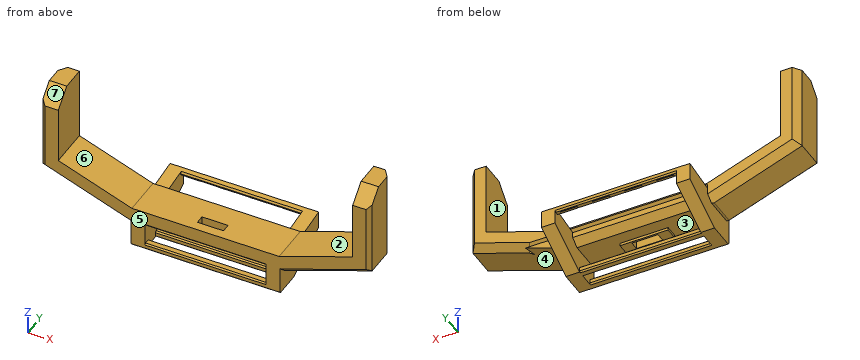
```python
from build123d import *
from OCP.BRepFilletAPI import BRepFilletAPI_MakeChamfer

# Parameters (mm, degrees)
BOSS_EXTRUDE1_DEPTH      = 300
CHAMFER1_SIZE            = 30
CHAMFER2_SIZE            = 120
BOSS_EXTRUDE2_DEPTH      = 180
BOSS_EXTRUDE2_DEPTH_BACK = 120
SKETCH3_W                = 101.940118113
SKETCH3_H                = 551.842685694
CUT_EXTRUDE7_DEPTH       = 1991.965553697
CHAMFER3_SIZE            = 170
CHAMFER3_SIZE2           = 348.551653068
SKETCH6_W                = 46.442322401
SKETCH6_H                = 54.989404456
SKETCH6_H_2              = 57.655849519
BOSS_EXTRUDE3_DEPTH      = 906.440509715
CHAMFER5_SIZE            = 10
CHAMFER5_SIZE2           = 11.720638091
SKETCH7_W                = 359.809632682
SKETCH7_H                = 90.64577865
BOSS_EXTRUDE4_DEPTH      = 20
SKETCH8_W                = 195
SKETCH8_H                = 65
CUT_EXTRUDE8_DEPTH       = 392
SKETCH9_W                = 124.341085276
SKETCH9_H                = 16.237188454
BOSS_EXTRUDE5_DEPTH      = 5
CHAMFER6_SIZE            = 60
CHAMFER6_SIZE2           = 43.59255168


with BuildPart() as part:
    # Sketch2 → Boss-Extrude1 (new body)
    with BuildSketch(Plane(origin=(0, 0, 0), x_dir=(1, 0, 0), z_dir=(0, 1, 0))):
        Polygon((-1100, -366.154475502), (-1100, 177.470675031), (-550, 377.470675031), (550, 377.470675031), (1100, 177.470675031), (1100, -377.470675031), (1230, -377.470675031), (1230, 268.52621943), (572.902747098, 507.470675031), (-572.902747098, 507.470675031), (-1230, 268.52621943), (-1230, -366.154475502), align=None)
    extrude(amount=BOSS_EXTRUDE1_DEPTH)

    # Chamfer1
    chamfer1_edges = [part.edges().sort_by_distance(p)[0] for p in [
        (-1230, 0, 48.814128036),
        (-901.451373549, 0, -387.99844723),
        (0, 0, -507.470675031),
        (901.451373549, 0, -387.99844723),
        (1230, 0, 54.4722278),
    ]]
    chamfer(chamfer1_edges, length=CHAMFER1_SIZE)

    # Chamfer2
    chamfer2_edges = [part.edges().sort_by_distance(p)[0] for p in [
        (-1150, 0, 366.154475502),
        (1150, 0, 377.470675031),
    ]]
    chamfer(chamfer2_edges, length=CHAMFER2_SIZE)

    # Sketch3 → Boss-Extrude2 (add, two sides: drawn at the far end of the back side and taken through both)
    with BuildSketch(Plane(origin=(0, 0, -507.470675031), x_dir=(-1, 0, 0), z_dir=(0, 0, -1)).offset(-BOSS_EXTRUDE2_DEPTH_BACK)):
        with Locations((-504.190313915, 275.921342847)):
            Rectangle(SKETCH3_W, SKETCH3_H)
        with Locations((504.190313915, 275.921342847)):
            Rectangle(SKETCH3_W, SKETCH3_H)
    extrude(amount=BOSS_EXTRUDE2_DEPTH + BOSS_EXTRUDE2_DEPTH_BACK)

    # Sketch5 → Cut-Extrude7 (cut, through all)
    with BuildSketch(Plane.ZY.offset(555.160372971)):
        Polygon((-387.470675031, 551.842685694), (-433.497227826, 219.864084998), (-387.470675031, 300), align=None)
    extrude(amount=-CUT_EXTRUDE7_DEPTH, mode=Mode.SUBTRACT)

    # Chamfer3: one chamfer whose edges measure the first distance from different faces: ONE call of the kernel's chamfer builder (chamfer() names one face for all edges)
    chamfer3_edges_1 = [part.edges().sort_by_distance(p)[0] for p in [
        (-504.190313915, 551.842685694, -687.470675031),
    ]]
    chamfer3_side_1 = [part.faces().sort_by_distance(p)[0] for p in [
        (-504.190313915, 551.842685694, -537.470675031),
    ]]
    chamfer3_edges_2 = [part.edges().sort_by_distance(p)[0] for p in [
        (504.190313915, 551.842685694, -687.470675031),
    ]]
    chamfer3_side_2 = [part.faces().sort_by_distance(p)[0] for p in [
        (504.190313915, 551.842685694, -537.470675031),
    ]]
    chamfer3 = BRepFilletAPI_MakeChamfer(part.part.solid().wrapped)
    for e in chamfer3_edges_1:
        chamfer3.Add(CHAMFER3_SIZE, CHAMFER3_SIZE2, e.wrapped, chamfer3_side_1[0].wrapped)  # the first distance lies on this face
    for e in chamfer3_edges_2:
        chamfer3.Add(CHAMFER3_SIZE, CHAMFER3_SIZE2, e.wrapped, chamfer3_side_2[0].wrapped)  # the first distance lies on this face
    add(Compound.cast(chamfer3.Shape()), mode=Mode.REPLACE)

    # Sketch6 → Boss-Extrude3 (add)
    with BuildSketch(Plane(origin=(-453.220254858, 0, 0), x_dir=(0, 0, -1), z_dir=(1, 0, 0))):
        Polygon((387.470675031, 551.842685694), (393.758008235, 506.493643621), (421.699837769, 506.493643621), (421.699837769, 551.842685694), align=None)
        with Locations((664.249513831, 175.796330397)):
            Rectangle(SKETCH6_W, SKETCH6_H)
        with Locations((664.249513831, 28.82792476)):
            Rectangle(SKETCH6_W, SKETCH6_H_2)
    extrude(amount=BOSS_EXTRUDE3_DEPTH)

    # Chamfer5: one chamfer whose edges measure the first distance from different faces: ONE call of the kernel's chamfer builder (chamfer() names one face for all edges)
    chamfer5_edges_1 = [part.edges().sort_by_distance(p)[0] for p in [
        (0, 506.493643621, -421.699837769),
        (0, 551.842685694, -421.699837769),
        (0, 148.301628169, -641.02835263),
        (0, 203.291032625, -641.02835263),
        (0, 203.291032625, -687.470675031),
        (0, 148.301628169, -687.470675031),
        (0, 0, -641.02835263),
        (0, 57.655849519, -641.02835263),
        (0, 57.655849519, -687.470675031),
        (0, 0, -687.470675031),
    ]]
    chamfer5_edges_2 = [part.edges().sort_by_distance(p)[0] for p in [
        (0, 506.493643621, -393.758008235),
    ]]
    chamfer5_side_2 = [part.faces().sort_by_distance(p)[0] for p in [
        (-541.133646758, 425.921342847, -404.928804327),
    ]]
    chamfer5 = BRepFilletAPI_MakeChamfer(part.part.solid().wrapped)
    for e in chamfer5_edges_1:
        chamfer5.Add(CHAMFER5_SIZE, e.wrapped)
    for e in chamfer5_edges_2:
        chamfer5.Add(CHAMFER5_SIZE, CHAMFER5_SIZE2, e.wrapped, chamfer5_side_2[0].wrapped)  # the first distance lies on this face
    add(Compound.cast(chamfer5.Shape()), mode=Mode.REPLACE)

    # Sketch7 → Boss-Extrude4 (add)
    with BuildSketch(Plane(origin=(0, 0, -507.470675031), x_dir=(-1, 0, 0), z_dir=(0, 0, -1))):
        with Locations((0, 102.978738844)):
            Rectangle(SKETCH7_W, SKETCH7_H)
    extrude(amount=BOSS_EXTRUDE4_DEPTH)

    # Sketch8 → Cut-Extrude8 (cut)
    with BuildSketch(Plane(origin=(0, 0, -527.470675031), x_dir=(-1, 0, 0), z_dir=(0, 0, -1))):
        with Locations((0, 102.978738844)):
            Rectangle(SKETCH8_W, SKETCH8_H)
    extrude(amount=-CUT_EXTRUDE8_DEPTH, mode=Mode.SUBTRACT)

    # Sketch9 → Boss-Extrude5 (add)
    with BuildSketch(Plane(origin=(0, 0, -421.699837769), x_dir=(-1, 0, 0), z_dir=(0, 0, -1))):
        with Locations((-358.63050058, 528.640825731)):
            Rectangle(SKETCH9_W, SKETCH9_H)
        with Locations((-118.63050058, 528.640825731)):
            Rectangle(SKETCH9_W, SKETCH9_H)
        with Locations((121.36949942, 528.640825731)):
            Rectangle(SKETCH9_W, SKETCH9_H)
        with Locations((361.36949942, 528.640825731)):
            Rectangle(SKETCH9_W, SKETCH9_H)
    extrude(amount=BOSS_EXTRUDE5_DEPTH)

    # Chamfer6: one chamfer whose edges measure the first distance from different faces: ONE call of the kernel's chamfer builder (chamfer() names one face for all edges)
    chamfer6_edges_1 = [part.edges().sort_by_distance(p)[0] for p in [
        (-1230, 300, 48.814128036),
    ]]
    chamfer6_side_1 = [part.faces().sort_by_distance(p)[0] for p in [
        (-1230, 167.541631542, 41.858763366),
    ]]
    chamfer6_edges_2 = [part.edges().sort_by_distance(p)[0] for p in [
        (-901.451373549, 300, -387.99844723),
    ]]
    chamfer6_side_2 = [part.faces().sort_by_distance(p)[0] for p in [
        (-901.451373549, 165, -387.99844723),
    ]]
    chamfer6_edges_3 = [part.edges().sort_by_distance(p)[0] for p in [
        (0, 300, -507.470675031),
    ]]
    chamfer6_side_3 = [part.faces().sort_by_distance(p)[0] for p in [
        (0, 174.536120756, -507.470675031),
    ]]
    chamfer6_edges_4 = [part.edges().sort_by_distance(p)[0] for p in [
        (1066.451373549, 300, -327.99844723),
    ]]
    chamfer6_side_4 = [part.faces().sort_by_distance(p)[0] for p in [
        (903.063859392, 162.599697247, -387.412088742),
    ]]
    chamfer6_edges_5 = [part.edges().sort_by_distance(p)[0] for p in [
        (1230, 300, 54.4722278),
    ]]
    chamfer6_side_5 = [part.faces().sort_by_distance(p)[0] for p in [
        (1230, 167.496050319, 47.507095726),
    ]]
    chamfer6 = BRepFilletAPI_MakeChamfer(part.part.solid().wrapped)
    for e in chamfer6_edges_1:
        chamfer6.Add(CHAMFER6_SIZE, CHAMFER6_SIZE2, e.wrapped, chamfer6_side_1[0].wrapped)  # the first distance lies on this face
    for e in chamfer6_edges_2:
        chamfer6.Add(CHAMFER6_SIZE, CHAMFER6_SIZE2, e.wrapped, chamfer6_side_2[0].wrapped)  # the first distance lies on this face
    for e in chamfer6_edges_3:
        chamfer6.Add(CHAMFER6_SIZE, CHAMFER6_SIZE2, e.wrapped, chamfer6_side_3[0].wrapped)  # the first distance lies on this face
    for e in chamfer6_edges_4:
        chamfer6.Add(CHAMFER6_SIZE, CHAMFER6_SIZE2, e.wrapped, chamfer6_side_4[0].wrapped)  # the first distance lies on this face
    for e in chamfer6_edges_5:
        chamfer6.Add(CHAMFER6_SIZE, CHAMFER6_SIZE2, e.wrapped, chamfer6_side_5[0].wrapped)  # the first distance lies on this face
    add(Compound.cast(chamfer6.Shape()), mode=Mode.REPLACE)


solid = part.part
```
Geometry: final body of the model. Coordinates: model frame, mm. Face numbers are marked on the shaded views. A direction names the side the tool comes from. Round coordinates to 2 decimals unless told otherwise and drop trailing zeros. Loops run counter-clockwise (first coordinate to the right, second up) from the corner with the lowest first, then second, coordinate; pieces in that order, holes last. Notation, with made-up numbers: (7.25, -8.75) -> (40.25, -8.75) arc R32 cw to (40.25, 27.25) -> close; hole circle Ø8 at (-22, 11). An arc over 180 degrees is marked (long way). Use one line per item in the form item = value. Start each with the question number.
1) Section A-A on z = -562. Output: boundary loops of the cut face in (x, y).
2) Draft query along Z for the marked faces 1, 2, 3 and 4. Return one class per face: released by +Z, released by -Z, zero draft, split by the parting line, or undercut.
3) First-contact query: P1, Ø2, axis at x = -396, y = 258.5, coming from the +Z side; P2, Ø21, axis at x = -173, z = -660.5, coming from the +Y side; P3, Ø4, axis at y = 528, z = -423.5, coming from the +X side; P4, Ø4, axis at x = -130, z = -424.5, coming from the -Y side. Flat tips, straight axial feed; report the tip coordinate or a pass-through.
4) Section C-C on x = 379.5. Give the number of separate pieces and of enclosed holes in the cut face, then the cut area to 3 significant figures.
5) Section B-B on y = 349.5. Output: boundary loops of the cut face in (x, z).
6) Line query: L1, parallel to X at y = 251.5, z = -606.5; L2, parallel to X at y = 74.5, z = 19; L3, parallel to Z at x = -365.5, y = 126.5. Output: solid intervals per line, ascending.
7) Access query for the marked faces 5, 6 and 7. Directions: +Z, -Z, +X, -X, +Y, -Y. A direction counts if a zero-diameter tool reaches every point of the face in a straight line with its end or side. Return the directions, or none.
8) Section D-D on x = -922.5. Output: boundary loops of the cut face in (y, z), then the cut area to 3 significant figures.
Response:
q1.outline = (-555.16, 0) -> (-453.22, 0) -> (-453.22, 460.54) -> (-555.16, 460.54) -> close; (453.22, 0) -> (555.16, 0) -> (555.16, 460.54) -> (453.22, 460.54) -> close
q2.face_1 = zero draft
q2.face_2 = released by +Z
q2.face_3 = undercut
q2.face_4 = released by -Z
q3.P1 = -377.47
q3.P2 = 203.29
q3.P3 = 555.16
q3.P4 = 0
q4.separate_pieces = 4
q4.enclosed_holes = 0
q4.area = 42,000 mm^2
q5.outline = (-555.16, -616.16) -> (-453.22, -616.16) -> (-453.22, -415.52) -> (-555.16, -415.52) -> close; (453.22, -616.16) -> (555.16, -616.16) -> (555.16, -415.52) -> (453.22, -415.52) -> close
q6.L1 = -555.16 to -453.22, 453.22 to 555.16
q6.L2 = -1230 to -1100, 1100 to 1230
q6.L3 = -507.47 to -377.47
q7.face_5 = +Z, -Z, +X, -X, -Y
q7.face_6 = +Z, +Y, -Y
q7.face_7 = +Z, -X, -Y
q8.outline = (0, -348.42) -> (30, -380.34) -> (240, -380.34) -> (300, -333.96) -> (300, -242.02) -> (0, -242.02) -> close
q8.area = 39,600 mm^2
